from build123d import *

# Parameters (mm, degrees)
BOSS_EXTRUDE1_DEPTH       = 8.89
SKETCH2_3_R               = 21.805
CUT_EXTRUDE1_DEPTH        = 3.2
ADVANCEDHOLE1_START       = 3.556
ADVANCEDHOLE1_OUTLINE_R   = 5
ADVANCEDHOLE1_DEPTH       = 5.334
ADVANCEDHOLE1_2_OUTLINE_R = 2.75
ADVANCEDHOLE1_2_DEPTH     = 3.556
SKETCH12_R                = 15.75
CUT_EXTRUDE2_DEPTH        = 3.2
ADVANCEDHOLE5_OUTLINE_R   = 3
ADVANCEDHOLE5_DEPTH       = 8.89
M6X1_0_TAPPED_HOLE1_D     = 6


# Read off the part's stored shape, not the designer's step: AdvancedHole1, AdvancedHole5
with BuildPart() as part:
    # Sketch2 → Boss-Extrude1 (new body)
    with BuildSketch(Plane.XY):
        Polygon((-13.151280605, 31.75), (-31.75, 13.151280605), (-31.75, -13.151280605), (-13.151280605, -31.75), (13.151280605, -31.75), (31.75, -13.151280605), (31.75, 13.151280605), (13.151280605, 31.75), align=None)
    extrude(amount=BOSS_EXTRUDE1_DEPTH)

    # Sketch2<3> → Cut-Extrude1 (cut)
    with BuildSketch(Plane.XY):
        Circle(SKETCH2_3_R)
    extrude(amount=CUT_EXTRUDE1_DEPTH, mode=Mode.SUBTRACT)

    # AdvancedHole1 outline → AdvancedHole1 (cut)
    with BuildSketch(Plane.XY.offset(ADVANCEDHOLE1_START)):
        with Locations((-25.76, 0)):
            Circle(ADVANCEDHOLE1_OUTLINE_R)
        with Locations((0, -25.76)):
            Circle(ADVANCEDHOLE1_OUTLINE_R)
        with Locations((25.76, 0)):
            Circle(ADVANCEDHOLE1_OUTLINE_R)
        with Locations((0, 25.76)):
            Circle(ADVANCEDHOLE1_OUTLINE_R)
    extrude(amount=ADVANCEDHOLE1_DEPTH, mode=Mode.SUBTRACT)

    # AdvancedHole1 2 outline → AdvancedHole1 2 (cut)
    with BuildSketch(Plane.XY):
        with Locations((-25.76, 0)):
            Circle(ADVANCEDHOLE1_2_OUTLINE_R)
        with Locations((0, -25.76)):
            Circle(ADVANCEDHOLE1_2_OUTLINE_R)
        with Locations((25.76, 0)):
            Circle(ADVANCEDHOLE1_2_OUTLINE_R)
        with Locations((0, 25.76)):
            Circle(ADVANCEDHOLE1_2_OUTLINE_R)
    extrude(amount=ADVANCEDHOLE1_2_DEPTH, mode=Mode.SUBTRACT)

    # Sketch12 → Cut-Extrude2 (cut)
    with BuildSketch(Plane.XY.offset(8.89)):
        Circle(SKETCH12_R)
    extrude(amount=-CUT_EXTRUDE2_DEPTH, mode=Mode.SUBTRACT)

    # AdvancedHole5 outline → AdvancedHole5 (cut)
    with BuildSketch(Plane.XY):
        with Locations((23.096988313, -9.567085809)):
            Circle(ADVANCEDHOLE5_OUTLINE_R)
    extrude(amount=ADVANCEDHOLE5_DEPTH, mode=Mode.SUBTRACT)

    # M6x1.0 Tapped Hole1 (through all)
    with Locations(Plane(origin=(-9.567085809, 23.096988313, 0), x_dir=(-1, 0, 0), z_dir=(0, 0, -1))):
        with Locations((0, 0), (-32.664074122, -13.529902504), (-19.134171618, -46.193976626), (13.529902504, -32.664074122)):
            Hole(M6X1_0_TAPPED_HOLE1_D / 2)


solid = part.part
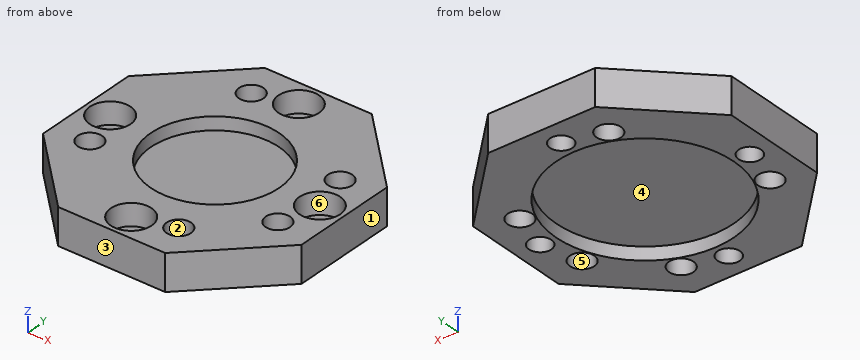
Build history of the part. All positions in model axes, mm. Face numbers are marked on the shaded views. A direction names the side the tool comes from. Round coordinates to 2 decimals unless told otherwise and drop trailing zeros. Write each loop counter-clockwise with the first axis right and the second up, starting at its lowest first coordinate (ties: lowest second). Pieces come first, ordered by that corner, then holes. Notation, with made-up numbers: M 54,81 L 63,81 A22 ccw 63,119 Z; hole C -12,30 d9. An arc over 180 degrees is marked long. Use CSV: the item, a comma, the result in double quotes.
1. Two-plate mould, pull along Y, no slides. Class the marked faces 1, 2 and 3: +Y half, -Y half, draft (parallel to the pull), parting line (faces both ways), or undercut.
Reply:
face 1,"draft"
face 2,"undercut"
face 3,"-Y half"
2. Tool access for the marked faces 4, 5 and 6: list every direction of +Z, -Z, +X, -X, +Y, -Y with a clear straight run to the whole face (end or side of a thin tool).
Reply:
face 4,"-Z"
face 5,"+Z, -Z"
face 6,"+Z"
3. Saw through at A-A (y = 0). Give the cut face in (x, z) (3 decimals), plus the area to 3 significant figures.
Reply:
outline,"M -31.75,0 L -28.51,0 L -28.51,3.556 L -30.76,3.556 L -30.76,8.89 L -31.75,8.89 Z; M -23.01,0 L -21.805,0 L -21.805,3.2 L 21.805,3.2 L 21.805,0 L 23.01,0 L 23.01,3.556 L 20.76,3.556 L 20.76,8.89 L 15.75,8.89 L 15.75,5.69 L -15.75,5.69 L -15.75,8.89 L -20.76,8.89 L -20.76,3.556 L -23.01,3.556 Z; M 28.51,0 L 31.75,0 L 31.75,8.89 L 30.76,8.89 L 30.76,3.556 L 28.51,3.556 Z"
area,"178 mm²"
4. Flat gauge pins, fed straight in: pin 1 (9 mm diameter, centred on x = 25.76, y = 0, fed in from -Z); pin 2 (19 mm diameter, centred on x = 0, y = 0, fed in from +Z); pin 3 (3 mm diameter, centred on x = -19, z = 3.5, fed in from -Y); pin 4 (22 mm diameter, centred on x = 1, y = -5.5, fed in from -Z). Where does each tip first touch, or does it go through?
Reply:
pin 1,"stops at z = 0"
pin 2,"stops at z = 5.69"
pin 3,"stops at y = -27.4"
pin 4,"stops at z = 3.2"
5. Saw through at D-D (x = -18.5). Give the cut face in (y, z), plus the area to 3 significant figures.
Reply:
outline,"M -26.4,0 L -11.54,0 L -11.54,3.2 L 11.54,3.2 L 11.54,0 L 26.4,0 L 26.4,8.89 L -26.4,8.89 Z"
area,"396 mm²"
6. Wall check: probe 1 along Y at (x, z) = (0, 5.45); probe 2 along Y at (x, z) = (0, 1.7) (3 decimals); probe 3 along Y at (x, z) = (-9, 7.5). Give the ranges that are in metal, low to high. Write a range as from..to.
Reply:
probe 1,"y = -31.75..-30.76, -20.76..20.76, 30.76..31.75"
probe 2,"y = -31.75..-28.51, -23.01..-21.805, 21.805..23.01, 28.51..31.75"
probe 3,"y = -31.75..-12.93, 12.93..20.15, 26.04..31.75"
7. Saw through at C-C (y = 15). Give the cut face in (x, z).
Reply:
outline,"M -29.9,0 L -15.83,0 L -15.83,3.2 L 15.83,3.2 L 15.83,0 L 29.9,0 L 29.9,8.89 L 4.8,8.89 L 4.8,5.69 L -4.8,5.69 L -4.8,8.89 L -29.9,8.89 Z"
